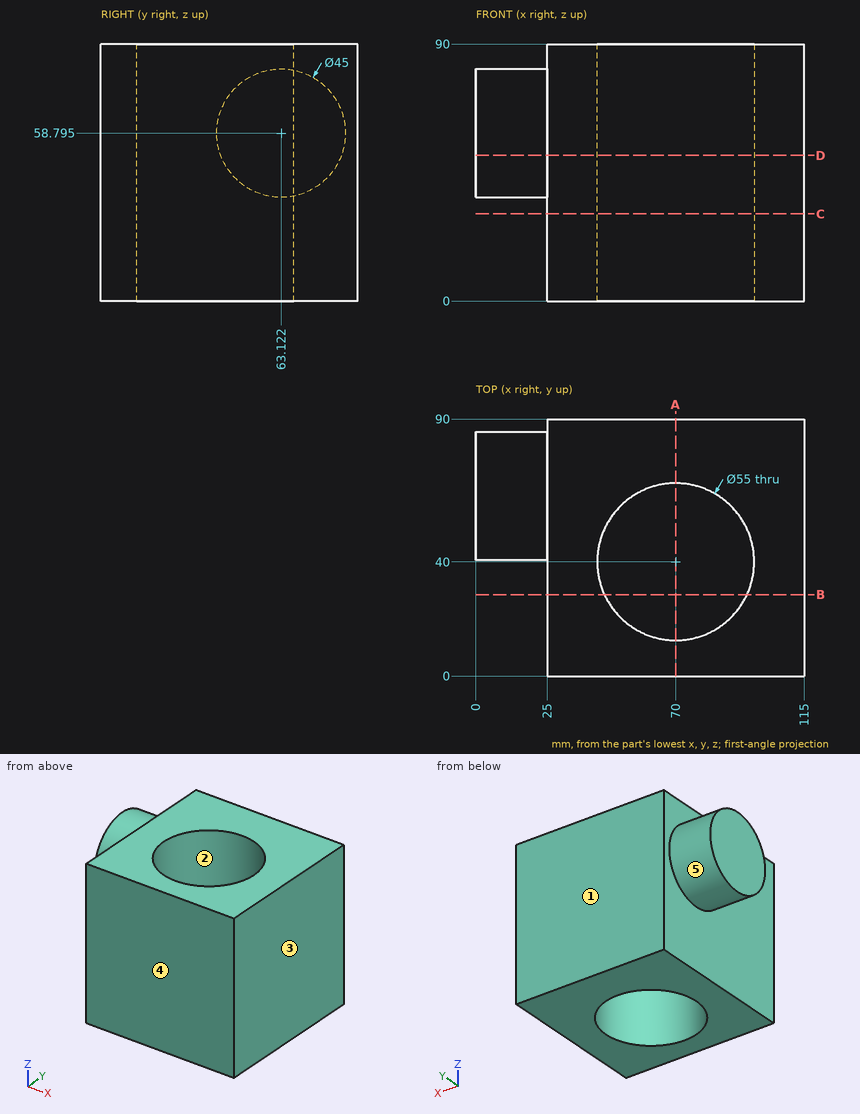
The figure shows three views and two pictorial views of one solid part (mm, origin at its lowest corner). Answer the questions. A direction names the side the tool comes from. Coordinates: 2 decimals unless noted, no trailing zeros. Order: outer loops, then holes, each group sorted by start corner. A loop starts at its lowest first (then second) coordinate and runs counter-clockwise, first axis right, second up.
Q1. For a pull along X with two mould halves and no side action, classify the marked faces 1, 2 and 3 as pulls with the +X half, pulls with the -X half, needs draft (parallel to the pull), parting line crosses it, or undercut.
Q2. Consider line 1 (Y direction, x = 70, z = 46.5); line 2 (X direction, y = 39.5, z = 54) (1 decimal); line 3 (X direction, y = 14.5, z = 40) (1 decimal). Determine where each line is inside the solid, lowest interval first.
Q3. Which of the six approach directions +Z, -Z, +X, -X, +Y, -Y give full straight-line access (tool end or side, diameter ignored) to the marked faces 4 and 5?
Q4. A cutting plane is placed at A-A, the plane x = 70. Write down the section's boundary in (y, z).
Q5. A cutting plane is placed at C-C, the plane z = 30.5. Write down the section's boundary in (x, y), and give its area (3 significant figures).
Q6. A cutting plane is placed at B-B, the plane y = 28.5. Write down the section's boundary in (x, z), and give its area (3 significant figures).
Q7. A cutting plane is placed at D-D, the plane z = 51. Write down the section's boundary in (x, y) (1 decimal).
Answers follow:
1. face 1: needs draft
1. face 2: undercut
1. face 3: pulls with the +X half
2. line 1: y = 0 to 12.5, 67.5 to 90
2. line 2: x = 25 to 42.5, 97.5 to 115
2. line 3: x = 25 to 59.7, 80.3 to 115
3. face 4: +Z, -Z, +X, -X, -Y
3. face 5: -X
4. outline: (0, 0) - (12.5, 0) - (12.5, 90) - (0, 90) - close; (67.5, 0) - (90, 0) - (90, 90) - (67.5, 90) - close
5. outline: (25, 0) - (115, 0) - (115, 90) - (25, 90) - close; hole circle Ø55 at (70, 40)
5. area: 5,720 mm2
6. outline: (25, 0) - (45.02, 0) - (45.02, 90) - (25, 90) - close; (94.98, 0) - (115, 0) - (115, 90) - (94.98, 90) - close
6. area: 3,600 mm2
7. outline: (0, 42) - (25, 42) - (25, 0) - (115, 0) - (115, 90) - (25, 90) - (25, 84.2) - (0, 84.2) - close; hole circle Ø55 at (70, 40)
